The listing builds one solid part. Answer for the finished solid, in the listing's coordinates (mm). A direction names the side the tool comes from. Round coordinates to 2 decimals unless told otherwise and drop trailing zeros. Write each loop counter-clockwise with the first axis right and the second up, starting at its lowest first coordinate (ties: lowest second). Pieces come first, ordered by that corner, then holes. Notation, with made-up numbers: (21, -30.75) - (58, -30.75) arc R27 cw to (58, -5.75) - close; hole circle Ø9 at (87.25, 2.25). An arc over 180 degrees is marked (long way). Answer as CSV lines item,"result". Start each with the question number.
Item 1: For a pull along Z with two mould halves and no side action, classify faces 3 (the flat face through (49, -60, 22)), 4 (the flat face through (46, -59, 45)), 5 (the cylindrical face through (33.44, -1.48, 30.44)) as pulls with the +Z half, pulls with the -Z half, needs draft (parallel to the pull), parting line crosses it, or undercut.
Item 2: A cutting plane is placed at C-C on x = 47.5. Determine the outline of the cut face in (y, z), and give its area (3 significant figures).
Item 3: Straight lines are drawn through the part: line 1 along X through (y, z) = (-27, 9.5); line 2 along Y through (x, z) = (43, 42.5); line 3 along Z through (x, y) = (60.5, -11.5). For each, find the intervals that lie inside material, in ascending order. Write a range as [from, to].
Item 4: A cutting plane is placed at A-A on z = 5.5. Determine the outline of the cut face in (x, y), and give its area (3 significant figures).
Item 5: A cutting plane is placed at D-D on y = -42. Determine the outline of the cut face in (x, z).
Item 6: Flat-ended cylindrical pins translate along their axes: pin 1 (1.5 mm diameter, centred on x = 63, y = -7.5, fed in from +Z); pin 2 (21 mm diameter, centred on x = 50.27, z = 25.14, fed in from +Y). Find the tip coordinate at first contact, or state that the pin passes through.
Item 7: Which of the six approach directions +Z, -Z, +X, -X, +Y, -Y give full straight-line access (tool end or side, diameter ignored) to faces 1 (the flat face through (49, -30, 3)), 2 (the flat face through (100, -30, 22))?
Item 8: A cutting plane is placed at B-B on x = 70. Determine the outline of the cut face in (y, z).
```python
from build123d import *

# Parameters (mm, degrees)
F0_W     = 100
F0_H     = 60
F1_DEPTH = 45
F2_W     = 94
F2_H     = 54
F3_DEPTH = 42
F4_R     = 3
F5_R     = 17.648561216
F6_DEPTH = 25


with BuildPart() as f1:
    # F0 (on Top) → F1 (new body)
    with BuildSketch(Plane.XY):
        with Locations((50, -30)):
            Rectangle(F0_W, F0_H)
    extrude(amount=F1_DEPTH)

    # F2 (on face) → F3 (cut, through all)
    with BuildSketch(Plane.XY.offset(45)):
        with Locations((50, -30)):
            Rectangle(F2_W, F2_H)
    extrude(amount=-F3_DEPTH, mode=Mode.SUBTRACT)

    # F4
    f4_edges = [f1.edges().sort_by_distance(p)[0] for p in [
        (100, -60, 22.5),
        (100, 0, 22.5),
        (0, 0, 22.5),
        (0, -60, 22.5),
    ]]
    fillet(f4_edges, radius=F4_R)

    # F5 (on face) → F6 (cut)
    with BuildSketch(Plane(origin=(0, 0, 0), x_dir=(-1, 0, 0), z_dir=(0, 1, 0))):
        with Locations((-50.2731017768, 25.1400116831)):
            Circle(F5_R)
    extrude(amount=-F6_DEPTH, mode=Mode.SUBTRACT)


solid = f1.part
```
Geometry says:
1,face 3,"needs draft"
1,face 4,"pulls with the +Z half"
1,face 5,"undercut"
2,outline,"(-60, 0) - (0, 0) - (0, 7.71) - (-3, 7.71) - (-3, 3) - (-57, 3) - (-57, 45) - (-60, 45) - close; (-3, 42.57) - (0, 42.57) - (0, 45) - (-3, 45) - close"
2,area,"327 mm^2"
3,line 1,"x = [0, 3], [97, 100]"
3,line 2,"y = [-60, -57], [-3, 0]"
3,line 3,"z = [0, 3]"
4,outline,"(0, -57) arc R3 ccw to (3, -60) - (97, -60) arc R3 ccw to (100, -57) - (100, -3) arc R3 ccw to (97, 0) - (3, 0) arc R3 ccw to (0, -3) - close; hole (3, -57) - (97, -57) - (97, -3) - (3, -3) - close"
4,area,"916 mm^2"
5,outline,"(0, 0) - (100, 0) - (100, 45) - (97, 45) - (97, 3) - (3, 3) - (3, 45) - (0, 45) - close"
6,pin 1,"stops at z = 3"
6,pin 2,"stops at y = -57"
7,face 1,"+Z"
7,face 2,"+Z, -Z, +X, +Y, -Y"
8,outline,"(-60, 0) - (0, 0) - (0, 45) - (-3, 45) - (-3, 3) - (-57, 3) - (-57, 45) - (-60, 45) - close"
